```python
from build123d import *

# Parameters (mm, degrees)
CYLINDER163_R     = 2.58
CYLINDER163_DEPTH = 29
CYLINDER161_R     = 72.517
CYLINDER161_DEPTH = 3
CYLINDER160_R     = 76.708
CYLINDER160_DEPTH = 3
CYLINDER162_R     = 3.02
CYLINDER162_DEPTH = 2
CYLINDER159_R     = 9
CYLINDER159_DEPTH = 21
CYLINDER158_R     = 20.635
CYLINDER158_DEPTH = 41.275
CYLINDER157_R     = 24
CYLINDER157_DEPTH = 3.175
CYLINDER164_R     = 2.28
CYLINDER164_DEPTH = 29
BOX_W             = 210.82
BOX_H             = 228.6
BOX_DEPTH         = 19.5


with BuildPart() as cylinder015:
    # Cylinder163 → Cylinder163 (new body)
    with BuildSketch(Plane(origin=(76, 35, 14), x_dir=(1, 0, 0), z_dir=(0, 0, 1))):
        Circle(CYLINDER163_R)
    extrude(amount=CYLINDER163_DEPTH)


with BuildPart() as cylinder013:
    # Cylinder161 → Cylinder161 (new body)
    with BuildSketch(Plane(origin=(105.41, 148, 17), x_dir=(1, 0, 0), z_dir=(0, 0, 1))):
        Circle(CYLINDER161_R)
    extrude(amount=CYLINDER161_DEPTH)


with BuildPart() as cut021:
    # Cylinder160 → Cylinder160 (new body)
    with BuildSketch(Plane(origin=(105.41, 148, 17), x_dir=(1, 0, 0), z_dir=(0, 0, 1))):
        Circle(CYLINDER160_R)
    extrude(amount=CYLINDER160_DEPTH)

    # Cut021: cut Cylinder013
    add(cylinder013.part, mode=Mode.SUBTRACT)


with BuildPart() as cylinder014:
    # Cylinder162 → Cylinder162 (new body)
    with BuildSketch(Plane(origin=(178.41, 148, 18), x_dir=(1, 0, 0), z_dir=(0, 0, 1))):
        Circle(CYLINDER162_R)
    extrude(amount=CYLINDER162_DEPTH)


with BuildPart() as cylinder011:
    # Cylinder159 → Cylinder159 (new body)
    with BuildSketch(Plane(origin=(105.41, 35, 0), x_dir=(1, 0, 0), z_dir=(0, 0, 1))):
        Circle(CYLINDER159_R)
    extrude(amount=CYLINDER159_DEPTH)


with BuildPart() as cylinder010:
    # Cylinder158 → Cylinder158 (new body)
    with BuildSketch(Plane.XY):
        Circle(CYLINDER158_R)
    extrude(amount=CYLINDER158_DEPTH)


with BuildPart() as cut020:
    # Cylinder157 → Cylinder157 (new body)
    with BuildSketch(Plane.XY):
        Circle(CYLINDER157_R)
    extrude(amount=CYLINDER157_DEPTH)

    # Cut020: cut Cylinder010
    add(cylinder010.part, mode=Mode.SUBTRACT)


with BuildPart() as cut020_1:
    # Cut020 placement: moved
    add(cut020.part.moved(Location((105.41, 35, 18.25))))


with BuildPart() as fusion058:
    # Cylinder164 → Cylinder164 (new body)
    with BuildSketch(Plane(origin=(135, 35, 14), x_dir=(1, 0, 0), z_dir=(0, 0, 1))):
        Circle(CYLINDER164_R)
    extrude(amount=CYLINDER164_DEPTH)

    # Fusion058: union Cylinder015, Cut021, Cylinder014, Cylinder011, Cut020
    add(cylinder015.part)
    add(cut021.part)
    add(cylinder014.part)
    add(cylinder011.part)
    add(cut020_1.part)


with BuildPart() as base_cut022:
    # Box → Box (new body)
    with BuildSketch(Plane.XY):
        with Locations((105.41, 114.3)):
            Rectangle(BOX_W, BOX_H)
    extrude(amount=BOX_DEPTH)

    # Cut022: cut Fusion058
    add(fusion058.part, mode=Mode.SUBTRACT)


solid = base_cut022.part
```
Model file for the job. Use its own axes, mm. A direction names the side the tool comes from. Coordinates: 2 decimals unless noted, no trailing zeros. One line per item, written item: value. Start each with the question number.
1. Tool access for faces 5 (the cylindrical face through (127.58, 25.81, 18.87)), 6 (the flat face through (104, 65, 19.5)): list every direction of +Z, -Z, +X, -X, +Y, -Y with a clear straight run to the whole face (end or side of a thin tool).
2. Probe line 1 (Y direction, x = 105.41, z = 19) (3 decimals); line 2 (Y direction, x = 76, z = 17.6); line 3 (X direction, y = 35, z = 18.9) (3 decimals). List the from-to ranges inside material, lowest first. Write a range as from..to.
3. Mould opens along Y. For faces 1 (the flat face through (104, 0, 10)), 2 (the flat face through (116, 53, 18.25)), 3 (the flat face through (162, 194, 17)), 4 (the flat face through (104, 149, 19.5)) say: released by +Y, released by -Y, zero draft, split by the parting line, or undercut.
4. Flat gauge pins, fed straight in: pin 1 (1.4 mm diameter, centred on x = 134.5, y = 34.5, fed in from +Z); pin 2 (2 mm diameter, centred on y = 127, z = 7.5, fed in from -X); pin 3 (11 mm diameter, centred on x = 105.41, y = 35, fed in from -Z); pin 4 (2 mm diameter, centred on x = 176.5, y = 148, fed in from +Z). Where does each tip first touch, or does it go through?
Answers below:
1. face 5: +Z
1. face 6: +Z, +X, -X, +Y, -Y
2. line 1: y = 0..11, 14.365..26, 44..55.635, 59..71.292, 75.483..220.517, 224.708..228.6
2. line 2: y = 0..32.42, 37.58..77.15, 81.71..214.29, 218.85..228.6
2. line 3: x = 0..73.42, 78.58..81.41, 84.775..96.41, 114.41..126.045, 129.41..132.72, 137.28..210.82
3. face 1: released by -Y
3. face 2: undercut
3. face 3: undercut
3. face 4: zero draft
4. pin 1: stops at z = 14
4. pin 2: stops at x = 0
4. pin 3: passes through
4. pin 4: stops at z = 18
